Build history of the part. All positions in model axes, mm. A direction names the side the tool comes from. Round coordinates to 2 decimals unless told otherwise and drop trailing zeros. Loops run counter-clockwise (first coordinate to the right, second up) from the corner with the lowest first, then second, coordinate; pieces in that order, holes last. Notation, with made-up numbers: M 16.5,-40 L 62.5,-40 A22 cw 62.5,-33 Z; hole C 13,-27 d10. An arc over 180 degrees is marked long. Write each question's results on one line, items separated by ' | '. Start each with the question number.
```python
from build123d import *

# Parameters (mm, degrees)
BOSS_EXTRUDE1_DEPTH  = 22.86
M3_CLEARANCE_HOLE1_D = 3.4


with BuildPart() as part:
    # Model → Boss-Extrude1 (new body)
    with BuildSketch(Plane.XY):
        Polygon((35.35946236, 21.996272555), (44.513095611, 15.400697433), (49.027368987, 9.071379605), (51.777733141, 1.917532085), (52.724150942, -5.518132067), (51.777733141, -12.953796218), (49.027368987, -20.107643738), (44.513095611, -26.436961567), (35.35946236, -33.032536689), (35.35946236, -56.318132067), (41.70946236, -56.318132067), (41.70946236, -36.283791365), (49.074837222, -30.976731111), (54.665181836, -23.138688335), (57.980059071, -14.51651143), (59.125380623, -5.518132067), (57.980059071, 3.480247297), (54.665181836, 12.102424201), (49.074837222, 19.940466977), (41.70946236, 25.247527231), (41.70946236, 45.281867933), (35.35946236, 45.281867933), align=None)
    extrude(amount=BOSS_EXTRUDE1_DEPTH)

    # M3 Clearance Hole1 (through all)
    with Locations(Plane(origin=(41.70946236, 0, 0), x_dir=(0, 0, -1), z_dir=(1, 0, 0))):
        with Locations((-17.78, 36.391867933), (-5.08, 36.391867933), (-17.78, -47.428132067), (-5.08, -47.428132067)):
            Hole(M3_CLEARANCE_HOLE1_D / 2)


solid = part.part
```
Item 1: Mould opens along Z. For faces 4 (the flat face through (50.4, 5.5, 11.3)), 5 (the cylindrical face through (38.49, 34.732, 17.411)), 6 (the flat face through (53, -9, 22.86)) say: released by +Z, released by -Z, zero draft, split by the parting line, or undercut.
Item 2: Saw through at C-C, the plane x = 43.5. Give the cut face in (y, z), then the cut area to 3 significant figures.
Item 3: Tool access for faces 1 (the flat face through (41.709, -46, 11)), 2 (the flat face through (52.244, -1.748, 11.27)), 3 (the flat face through (41.709, 35, 11)): list every direction of +Z, -Z, +X, -X, +Y, -Y with a clear straight run to the whole face (end or side of a thin tool).
Item 4: Drop flat-ended pins along their axis: pin 1 (5.5 mm diameter, centred on y = -47.43, z = 17.78, fed in from +X); pin 2 (4 mm diameter, centred on x = 44, z = 3.5, fed in from +Y); pin 3 (8 mm diameter, centred on x = 49.5, z = 8.5, fed in from +Y). Give the stop position or say it passes through.
Item 5: Drill centre lines: line 1 along Y through (x, z) = (37, 5.08); line 2 along Z through (x, y) = (38.5, -47); line 3 along Y through (x, z) = (38.5, 5.08). Where is each one in solid material? Low to high. Write a range as [from, to].
Item 6: Saw through at D-D, the plane z = 1.5. Give the cut face in (x, y), then the cut area to 3 significant figures.
Item 7: Saw through at A-A, the plane z = 17.78. State how many separate pieces and enclosed holes the cut face has, then the cut area to 3 significant figures.
Item 8: Saw through at B-B, the plane x = 37.5. Give the cut face in (y, z).
Working result:
1) face 4: zero draft | face 5: undercut | face 6: released by +Z
2) outline: M -34.99,0 L -27.17,0 L -27.17,22.86 L -34.99,22.86 Z; M 16.13,0 L 23.96,0 L 23.96,22.86 L 16.13,22.86 Z | area: 358 mm²
3) face 1: +Z, -Z, +X, -Y | face 2: +Z, -Z, -X | face 3: +Z, -Z, +X, +Y
4) pin 1: stops at x = 41.71 | pin 2: stops at y = 25.04 | pin 3: stops at y = 22.52
5) line 1: y = [-56.32, -49.13], [-45.73, -31.85], [20.81, 34.69], [38.09, 45.28] | line 2: z = [0, 3.43], [6.73, 16.13], [19.43, 22.86] | line 3: y = [-56.32, -49.13], [-45.73, -30.77], [19.73, 34.69], [38.09, 45.28]
6) outline: M 35.36,-56.32 L 41.71,-56.32 L 41.71,-36.28 L 49.07,-30.98 L 54.67,-23.14 L 57.98,-14.52 L 59.13,-5.52 L 57.98,3.48 L 54.67,12.1 L 49.07,19.94 L 41.71,25.25 L 41.71,45.28 L 35.36,45.28 L 35.36,22 L 44.51,15.4 L 49.03,9.07 L 51.78,1.92 L 52.72,-5.52 L 51.78,-12.95 L 49.03,-20.11 L 44.51,-26.44 L 35.36,-33.03 Z | area: 727 mm²
7) separate pieces: 3 | enclosed holes: 0 | area: 684 mm²
8) outline: M -56.32,0 L -31.49,0 L -31.49,22.86 L -56.32,22.86 Z; M 20.45,0 L 45.28,0 L 45.28,22.86 L 20.45,22.86 Z; hole C -47.43,5.08 d3.4; hole C -47.43,17.78 d3.4; hole C 36.39,5.08 d3.4; hole C 36.39,17.78 d3.4
